Read the model definition and answer for the solid it produces. Units are mm, in the model's axes. Face numbers are marked on the shaded views. A direction names the side the tool comes from. Coordinates: 2 decimals unless noted, no trailing zeros. Write each loop counter-clockwise with the first axis right and the second up, starting at its lowest first coordinate (ties: lowest second). Pieces come first, ordered by that corner, then holes. Notation, with made-up numbers: (-21, 48.5) -> (5, 48.5) arc R14 cw to (5, 73.5) -> close; hole circle Ø9 at (37, -6.5). An arc over 180 degrees is marked (long way). Use CSV: the item, a comma, the result in double quotes.
Autodesk Inventor part; units mm, degrees
ref_plane "Work Plane1" through (65, -5, 0) normal (-1, 0, 0) x (0, 0, 1)
ref_plane "YZ Plane" through (0, 0, 0) normal (1, 0, 0) x (0, 1, 0)
ref_plane "XZ Plane" through (0, 0, 0) normal (0, 1, 0) x (-1, 0, 0)
sketch "Sketch1" plane through (0, 0, 0) normal (0, 1, 0) x (-1, 0, 0)
  line L0 (0, 0) -> (-130, 0)
  line L1 (-130, 0) -> (-130, -100)
  line L2 (-130, -100) -> (0, -100)
  line L3 (0, -100) -> (0, 0)
  line L4 (-5, -21) -> (-57, -21) construction
  line L5 (-65, -21) -> (-65, -79) construction
  line L6 (-57, -79) -> (-5, -79) construction
  line L7 (-5, -79) -> (-5, -21) construction
  line L8 (-65, -91.7) -> (-120, -91.7) construction
  line L9 (-120, -91.7) -> (-120, -8.3) construction
  line L10 (-120, -8.3) -> (-65, -8.3) construction
  line L11 (-65, -8.3) -> (-65, -91.7) construction
  line L12 (-5, 0) -> (-5, -100)
  line L13 (-125, -100) -> (-125, 0)
  line L14 (-86.5, 0) -> (-98.5, 0)
  line L15 (-98.5, 0) -> (-98.5, -8.3)
  line L16 (-98.5, -8.3) -> (-86.5, -8.3)
  line L17 (-86.5, -8.3) -> (-86.5, 0)
  line L18 (-87.5, -100) -> (-97.5, -100)
  line L19 (-110, -93.2) -> (-120, -93.2)
  line L20 (-120, -93.2) -> (-120, -85.2)
  line L21 (-120, -85.2) -> (-125, -85.2)
  line L22 (-125, -85.2) -> (-125, -97.2)
  line L23 (-125, -97.2) -> (-110, -97.2)
  line L24 (-110, -97.2) -> (-110, -93.2)
  line L25 (-57, -79) -> (-57, -21) construction
  line L26 (-120, -8.3) -> (-105, -8.3)
  line L27 (-105, -8.3) -> (-105, -13.3)
  line L28 (-105, -13.3) -> (-120, -13.3)
  line L29 (-120, -13.3) -> (-120, -8.3)
  line L30 (-65, -8.3) -> (-80, -8.3)
  line L31 (-80, -8.3) -> (-80, -13.3)
  line L32 (-80, -13.3) -> (-65, -13.3)
  line L33 (-65, -13.3) -> (-65, -8.3)
  line L34 (-120, -91.7) -> (-105, -91.7)
  line L35 (-105, -91.7) -> (-105, -85.2)
  line L36 (-105, -85.2) -> (-120, -85.2)
  line L37 (-120, -85.2) -> (-120, -91.7)
  line L38 (-65, -91.7) -> (-80, -91.7)
  line L39 (-80, -91.7) -> (-80, -85.2)
  line L40 (-80, -85.2) -> (-65, -85.2)
  line L41 (-65, -85.2) -> (-65, -91.7)
  line L42 (-65, -42.5) -> (-60, -42.5)
  line L43 (-60, -42.5) -> (-60, -57.5)
  line L44 (-60, -57.5) -> (-65, -57.5)
  line L45 (-65, -57.5) -> (-65, -42.5)
  line L46 (-54, -75.75) -> (-8, -75.75) construction
  line L47 (-8, -75.75) -> (-8, -24.25) construction
  line L48 (-120, -91.7) -> (-105, -91.7)
  line L49 (-105, -91.7) -> (-105, -93.2)
  line L50 (-105, -93.2) -> (-120, -93.2)
  line L51 (-120, -93.2) -> (-120, -91.7)
  line L52 (-80, -91.7) -> (-65, -91.7)
  line L53 (-65, -91.7) -> (-65, -93.2)
  line L54 (-65, -93.2) -> (-80, -93.2)
  line L55 (-80, -93.2) -> (-80, -91.7)
  line L56 (-80, -93.2) -> (-65, -93.2)
  line L57 (-65, -93.2) -> (-65, -97.2)
  line L58 (-65, -97.2) -> (-80, -97.2)
  line L59 (-80, -97.2) -> (-80, -93.2)
  point P0 (0, -50)
  point P1 (-65, -50)
  point P2 (-65, -100)
  point P3 (-120, -50)
  point P4 (-120, -50)
  point P5 (-54, -24.25)
  point P6 (-92.5, -8.3)
  point P7 (-92.5, -8.3)
  point P8 (-86.5, 0)
  point P9 (-98.5, 0)
  point P10 (-45, -100)
  point P11 (-95, -100)
  point P12 (-92.5, -91.7)
  point P13 (-110, -95.2)
  point P14 (-115, -93.2)
  point P15 (-125, -85.2)
  point P16 (-125, -97.2)
  point P17 (-5, -50)
  point P18 (-57, -50)
  point P19 (-65, -50)
  point P20 (-31, -75.75)
  point P21 (-31, -79)
  point P22 (-8, -50)
  point P23 (-75, -93)
  point P24 (-65, -93)
  point P25 (-72.5, -97.2)
  point P26 (-65, -93.2)
  dimension "d0" = 100
  dimension "d1" = 130
  dimension "d2" = 52
  dimension "d3" = 58
  dimension "d5" = 55
  dimension "d6" = 83.4
  dimension "d10" = 5
  dimension "d11" = 5
  dimension "d16" = 12
  dimension "d17" = 8.3
  dimension "d88" = 10
  dimension "d89" = 5
  dimension "d90" = 4
  dimension "d92" = 8
  dimension "d93" = 1.5
  dimension "d101" = 15
  dimension "d102" = 15
  dimension "d103" = 6.5
  dimension "d104" = 5
  dimension "d105" = 15
  dimension "d111" = 0
  dimension "d112" = 15
  dimension "d113" = 5
  dimension "d116" = 46
  dimension "d117" = 51.5
extrude "Extrusion2" add sketch "Sketch1" against normal blind 5 contours L3 L2 L12 L0 | L12 L2 L13 L23 L24 L50 L49 L35 L36 L21 L0 L15 L16 L17 | L17 L16 L15 L0 | L13 L2 L1 L0 | L21 L20 L19 L24 L23 L13 | L36 L35 L34 L20 | L34 L49 L50 L19 L20 | L26 L27 L28 L29 | L33 L32 L31 L30 | L53 L54 L55 L38 | L38 L39 L40 L41 | L57 L58 L59 L54 | L42 L43 L44 L45
hole "Hole1" at (8, 0, -75.75) at (8, 0, -24.25) at (54, 0, -75.75) at (54, 0, -24.25) direction (0, -1, 0) diameter 3.1 end through all
extrude "Extrusion5" add sketch "Sketch1" along normal blind 50 contours L3 L2 L12 L0 | L13 L2 L1 L0
extrude "Extrusion6" add sketch "Sketch1" along normal blind 20 contours L17 L16 L15 L0 | L21 L20 L19 L24 L23 L13
ref_plane "Work Plane1" through (65, -5, 0) normal (-1, 0, 0) x (0, 0, 1)
sketch "Sketch5" plane through (0, -5, 0) normal (0, -1, 0) x (1, 0, 0)
  line L0 (130, 0) -> (0, 0)
  line L1 (65, 0) -> (65, -100)
  line L2 (0, -100) -> (130, -100)
  line L3 (5, -30) -> (10, -30)
  line L4 (10, -30) -> (10, -70)
  line L5 (10, -70) -> (5, -70)
  line L6 (5, -70) -> (5, -30)
  line L7 (125, -30) -> (120, -30)
  line L8 (120, -30) -> (120, -70)
  line L9 (120, -70) -> (125, -70)
  line L10 (125, -70) -> (125, -30)
  point P0 (65, -50)
  point P1 (10, -50)
  dimension "d60" = 40
  dimension "d61" = 5
  dimension "d62" = 55
extrude "Extrusion9" add sketch "Sketch5" along normal blind 15
sketch "Sketch6" plane through (5, -5, -70) normal (-1, 0, 0) x (0, 0, 1)
  line L0 (11.25, -6) -> (28.75, -6) construction
  line L1 (70, 0) -> (-30, 0)
  line L2 (11.25, 36) -> (28.75, 36)
  point P0 (70, 5)
  point P1 (20, 0)
  point P2 (20, -6)
  dimension "d65" = 17.5
  dimension "d66" = 6
  dimension "d74" = 17.5
hole "Hole2" at (5, -11, -58.75) at (5, -11, -41.25) direction (1, 0, 0) diameter 3.1 end through all
sketch "Sketch7" plane through (0, -5, -100) normal (-1, 0, 0) x (0, 0, 1)
  line L0 (41.25, 45) -> (58.75, 45) construction
  line L1 (100, 0) -> (0, 0)
  line L2 (0, 55) -> (100, 55)
  point P0 (100, 5)
  point P1 (50, 45)
  point P2 (50, 0)
  dimension "d75" = 17.5
  dimension "d76" = 10
hole "Hole3" at (0, 40, -58.75) at (0, 40, -41.25) direction (1, 0, 0) diameter 3.1 end through all
sketch "Sketch8" plane through (0, -5, -100) normal (-1, 0, 0) x (0, 0, 1)
  line L0 (100, 5) -> (0, 5)
  line L1 (15, 5) -> (85, 5)
  line L2 (85, 5) -> (85, 35)
  line L3 (85, 35) -> (15, 35)
  line L4 (15, 35) -> (15, 5)
  line L5 (0, 55) -> (100, 55)
  point P0 (14.8, 5)
  point P1 (50, 35)
  point P2 (50, 55)
  dimension "d95" = 70
  dimension "d96" = 30
extrude "Extrusion10" cut sketch "Sketch8" against normal through all
extrude "Extrusion11" add sketch "Sketch1" along normal blind 10 contours L36 L35 L34 L20 | L34 L49 L50 L19 L20 | L26 L27 L28 L29 | L33 L32 L31 L30 | L53 L54 L55 L38 | L38 L39 L40 L41
extrude "Extrusion13" add sketch "Sketch1" along normal blind 20 contours L57 L58 L59 L54 | L42 L43 L44 L45
properties part number "Chasis 2"
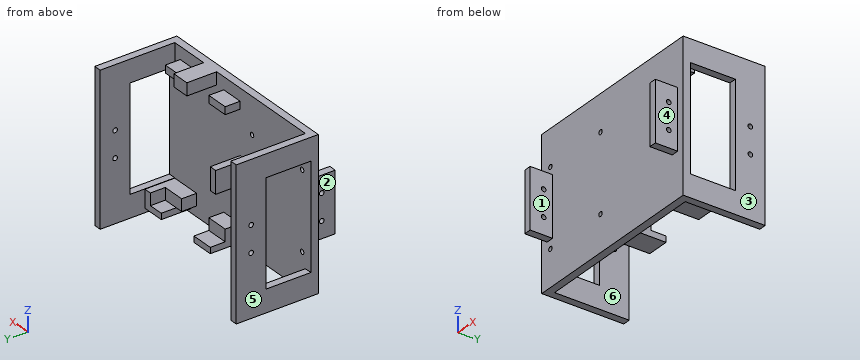
1. Each of these flat-tipped pins is pushed along its axis until it touches: pin 1 Ø8 at (x, y) = (109, 5) entering from +Z; pin 2 Ø5.5 at (x, y) = (127.5, 18) entering from +Z; pin 3 Ø12 at (x, z) = (100, -38) entering from -Y; pin 4 Ø1 at (x, z) = (86.5, -41.5) entering from +Y. Where does it stop, or does it pass through?
Solutions:
pin 1,"stops at z = -8.3"
pin 2,"stops at z = 0"
pin 3,"stops at y = -5"
pin 4,"stops at y = 0"
2. A cutting plane is placed at A-A (x = 8). Give the vertices of the cut face in (y, z).
Solutions:
outline,"(-20, -70) -> (-5, -70) -> (-5, -74.2) -> (0, -74.2) -> (0, -25.8) -> (-5, -25.8) -> (-5, -30) -> (-20, -30) -> close; (-5, -100) -> (0, -100) -> (0, -77.3) -> (-5, -77.3) -> close; (-5, -22.7) -> (0, -22.7) -> (0, 0) -> (-5, 0) -> close; hole circle Ø3.1 at (-11, -58.75); hole circle Ø3.1 at (-11, -41.25)"
3. Find the intervals of material crossed by line 1 along Y through (x, z) = (126.6, -41.25); line 2 along Z through (x, y) = (6, -11); line 3 along X through (y, z) = (-1, -24), in increasing order.
Solutions:
line 1,"y = -5 to 0, 30 to 38.45, 41.55 to 50"
line 2,"z = -70 to -60.3, -57.2 to -42.8, -39.7 to -30"
line 3,"x = 0 to 6.47, 9.53 to 52.47, 55.53 to 130"
4. A cutting plane is placed at B-B (z = -24.25). Give the vertices of the cut face in (x, y).
Solutions:
outline,"(0, -5) -> (6.45, -5) -> (6.45, 0) -> (0, 0) -> close; (0, 30) -> (5, 30) -> (5, 50) -> (0, 50) -> close; (9.55, -5) -> (52.45, -5) -> (52.45, 0) -> (9.55, 0) -> close; (55.55, -5) -> (130, -5) -> (130, 0) -> (55.55, 0) -> close; (125, 30) -> (130, 30) -> (130, 50) -> (125, 50) -> close"
5. A tool of negligible diameter and unlimited length cuts with its end or side. For the marked faces 4, 5 and 6, from which of +Z, -Z, +X, -X, +Y, -Y can it reach the whole face along a straight path? Write none if from no direction.
Solutions:
face 4,"+Z, -Z, +X, -Y"
face 5,"+Z, -Z, -X, +Y, -Y"
face 6,"+Z, -Z, +Y"
6. A cutting plane is placed at D-D (z = -36). Give the vertices of the cut face in (x, y), and give its area (3 significant figures).
Solutions:
outline,"(0, -5) -> (5, -5) -> (5, -20) -> (10, -20) -> (10, -5) -> (120, -5) -> (120, -20) -> (125, -20) -> (125, -5) -> (130, -5) -> (130, 0) -> (0, 0) -> close; (0, 30) -> (5, 30) -> (5, 50) -> (0, 50) -> close; (125, 30) -> (130, 30) -> (130, 50) -> (125, 50) -> close"
area,"1,000 mm^2"
7. For a pull along X with two mould halves and no side action, classify the marked faces 1, 2 and 3 as pulls with the +X half, pulls with the -X half, needs draft (parallel to the pull), parting line crosses it, or undercut.
Solutions:
face 1,"undercut"
face 2,"pulls with the -X half"
face 3,"pulls with the +X half"
8. A cutting plane is placed at C-C (y = -11). Give the vertices of the cut face in (x, z), and give its area (3 significant figures).
Solutions:
outline,"(5, -70) -> (10, -70) -> (10, -60.3) -> (5, -60.3) -> close; (5, -57.2) -> (10, -57.2) -> (10, -42.8) -> (5, -42.8) -> close; (5, -39.7) -> (10, -39.7) -> (10, -30) -> (5, -30) -> close; (120, -70) -> (125, -70) -> (125, -60.3) -> (120, -60.3) -> close; (120, -57.2) -> (125, -57.2) -> (125, -42.8) -> (120, -42.8) -> close; (120, -39.7) -> (125, -39.7) -> (125, -30) -> (120, -30) -> close"
area,"338 mm^2"
